```python
from build123d import *

# Parameters (mm, degrees)
CROQUIS1_R              = 5
SALIENTE_EXTRUIR1_DEPTH = 27
CROQUIS2_R              = 1.5
CORTAR_EXTRUIR1_DEPTH   = 5
CROQUIS4_R              = 1.5
CORTAR_EXTRUIR2_DEPTH   = 5


with BuildPart() as part:
    # Croquis1 → Saliente-Extruir1 (new body)
    with BuildSketch(Plane(origin=(0, 0, 0), x_dir=(1, 0, 0), z_dir=(0, 1, 0))):
        Circle(CROQUIS1_R)
    extrude(amount=SALIENTE_EXTRUIR1_DEPTH)

    # Croquis2 → Cortar-Extruir1 (cut)
    with BuildSketch(Plane(origin=(0, 27, 0), x_dir=(1, 0, 0), z_dir=(0, 1, 0))):
        Circle(CROQUIS2_R)
    extrude(amount=-CORTAR_EXTRUIR1_DEPTH, mode=Mode.SUBTRACT)

    # Croquis4 → Cortar-Extruir2 (cut)
    with BuildSketch(Plane.XZ):
        Circle(CROQUIS4_R)
    extrude(amount=-CORTAR_EXTRUIR2_DEPTH, mode=Mode.SUBTRACT)


solid = part.part
```
The listing builds one solid part. Answer for the finished solid, in the listing's coordinates (mm). A direction names the side the tool comes from. Round coordinates to 2 decimals unless told otherwise and drop trailing zeros. Write each loop counter-clockwise with the first axis right and the second up, starting at its lowest first coordinate (ties: lowest second). Pieces come first, ordered by that corner, then holes. Notation, with made-up numbers: (-20, 13.25) -> (21, 13.25) arc R22 ccw to (21, 19.25) -> close; hole circle Ø8 at (41, 76.25). An arc over 180 degrees is marked (long way). Use CSV: the item, a comma, the result in double quotes. Start each with the question number.
(1) Each of these flat-tipped pins is pushed along its axis until it touches: pin 1 (0.9 mm diameter, centred on x = -0.5, z = 0.5, fed in from +Y); pin 2 (1.5 mm diameter, centred on x = 0.5, z = 0.5, fed in from -Y); pin 3 (1.5 mm diameter, centred on x = -1.5, y = 22.5, fed in from -Z). Where does it stop, or does it pass through?
(2) Section A-A on y = 3.5 is taken. Give the vertices of the cut face in (x, z), then the cut area to 3 significant figures.
(3) The mould has two halves that part along Z. Classify faces 1 (the face through (-1.08, 13.31, 4.88)), 2 (the face through (-1.2, 0, -1.2)), 3 (the face through (-1.5, 24.54, -0.07)), 4 (the face through (0, 22, 0)): released by +Z, released by -Z, zero draft, split by the parting line, or undercut.
(4) Section B-B on x = 0 is taken. Give the vertices of the cut face in (y, z), then the cut area to 3 significant figures.
(5) Section C-C on z = 0 is taken. Give the vertices of the cut face in (x, y).
(6) Which of the six approach directions +Z, -Z, +X, -X, +Y, -Y give full straight-line access (tool end or side, diameter ignored) to faces 5 (the face through (-1.2, 27, -1.2)), 6 (the face through (0, 5, 0))?
(7) Section D-D on y = 13 is taken. Give the vertices of the cut face in (x, z).
(8) Consider L1, parallel to Z at x = 0, y = 24.95; L2, parallel to X at y = 11, z = 0.25. Determine where each line is inside the solid, lowest interval first. Write a range as from..to.
A:
1,pin 1,"stops at y = 22"
1,pin 2,"stops at y = 5"
1,pin 3,"stops at z = -4.94"
2,outline,"circle Ø10 at (0, 0); hole circle Ø3 at (0, 0)"
2,area,"71.5 mm²"
3,face 1,"split by the parting line"
3,face 2,"zero draft"
3,face 3,"undercut"
3,face 4,"undercut"
4,outline,"(0, -5) -> (27, -5) -> (27, -1.5) -> (22, -1.5) -> (22, 1.5) -> (27, 1.5) -> (27, 5) -> (0, 5) -> (0, 1.5) -> (5, 1.5) -> (5, -1.5) -> (0, -1.5) -> close"
4,area,"240 mm²"
5,outline,"(-5, 0) -> (-1.5, 0) -> (-1.5, 5) -> (1.5, 5) -> (1.5, 0) -> (5, 0) -> (5, 27) -> (1.5, 27) -> (1.5, 22) -> (-1.5, 22) -> (-1.5, 27) -> (-5, 27) -> close"
6,face 5,"+Z, -Z, +X, -X, +Y"
6,face 6,"-Y"
7,outline,"circle Ø10 at (0, 0)"
8,L1,"z = -5..-1.5, 1.5..5"
8,L2,"x = -4.99..4.99"
